Could you check a few things on this model? Use its own coordinates, in mm. A direction names the side the tool comes from. Round coordinates to 2 decimals unless told otherwise and drop trailing zeros. Loops run counter-clockwise (first coordinate to the right, second up) from the corner with the lowest first, then second, coordinate; pieces in that order, holes last. Notation, with made-up numbers: (27.5, 7) -> (74.5, 7) arc R9 cw to (74.5, 16) -> close; hole circle Ø9 at (65, 42). An arc over 180 degrees is marked (long way). Use CSV: the item, a comma, the result in double quotes. Start each with the question number.
```python
from build123d import *

# Parameters (mm, degrees)
BOSS_EXTRUDE1_DEPTH = 3
SKETCH3_W           = 10.2
SKETCH3_H           = 3.2
SKETCH3_W_2         = 3.2
SKETCH3_H_2         = 10.2
SKETCH3_H_3         = 7.372217102
CUT_EXTRUDE1_DEPTH  = 4


with BuildPart() as part:
    # Sketch2 → Boss-Extrude1 (new body)
    with BuildSketch(Plane(origin=(0, 0, 0), x_dir=(1, 0, 0), z_dir=(0, 1, 0))):
        with BuildLine():
            Line((-74.222217102, -66.842990858), (55.172217102, -66.842990858))
            Line((55.172217102, -66.842990858), (55.172217102, 43.501443346))
            Line((55.172217102, 43.501443346), (41.872217102, 43.501443346))
            ThreePointArc((41.872217102, 43.501443346), (38.336683196, 42.036977252), (36.872217102, 38.501443346))
            Line((36.872217102, 38.501443346), (36.872217102, -48.842990858))
            ThreePointArc((36.872217102, -48.842990858), (35.407751008, -52.378524764), (31.872217102, -53.842990858))
            Line((31.872217102, -53.842990858), (-31.872217102, -53.842990858))
            ThreePointArc((-31.872217102, -53.842990858), (-35.407751008, -52.378524764), (-36.872217102, -48.842990858))
            Line((-36.872217102, -48.842990858), (-36.872217102, 38.501443346))
            ThreePointArc((-36.872217102, 38.501443346), (-38.336683196, 42.036977252), (-41.872217102, 43.501443346))
            Line((-41.872217102, 43.501443346), (-74.222217102, 43.501443346))
            Line((-74.222217102, 43.501443346), (-74.222217102, -66.842990858))
        make_face()
    extrude(amount=-BOSS_EXTRUDE1_DEPTH)

    # Sketch3 → Cut-Extrude1 (cut, through all)
    with BuildSketch(Plane(origin=(0, 0, 0), x_dir=(1, 0, 0), z_dir=(0, 1, 0))):
        with Locations((-69.222217102, -65.342990858)):
            Rectangle(SKETCH3_W, SKETCH3_H)
        with Locations((-53.672217102, 18.329226244)):
            Rectangle(SKETCH3_W_2, SKETCH3_H_2)
        with Locations((-53.672217102, -1.670773756)):
            Rectangle(SKETCH3_W_2, SKETCH3_H_2)
        with Locations((-30, -65.342990858)):
            Rectangle(SKETCH3_W, SKETCH3_H)
        with Locations((-10, -65.342990858)):
            Rectangle(SKETCH3_W, SKETCH3_H)
        with Locations((-53.672217102, 36.915334795)):
            Rectangle(SKETCH3_W_2, SKETCH3_H_3)
        with Locations((30, -65.342990858)):
            Rectangle(SKETCH3_W, SKETCH3_H)
        with Locations((-53.672217102, -41.670773756)):
            Rectangle(SKETCH3_W_2, SKETCH3_H_2)
        with Locations((-53.672217102, -21.670773756)):
            Rectangle(SKETCH3_W_2, SKETCH3_H_2)
        with Locations((-53.672217102, -60.256882307)):
            Rectangle(SKETCH3_W_2, SKETCH3_H_3)
        Polygon((52.072217102, -56.570773756), (52.072217102, -63.742990858), (44.9, -63.742990858), (44.9, -66.942990858), (55.272217102, -66.942990858), (55.272217102, -56.570773756), align=None)
        with Locations((53.672217102, -21.670773756)):
            Rectangle(SKETCH3_W_2, SKETCH3_H_2)
        with Locations((53.672217102, -41.670773756)):
            Rectangle(SKETCH3_W_2, SKETCH3_H_2)
        with Locations((10, -65.342990858)):
            Rectangle(SKETCH3_W, SKETCH3_H)
        with Locations((53.672217102, 18.329226244)):
            Rectangle(SKETCH3_W_2, SKETCH3_H_2)
        with Locations((53.672217102, -1.670773756)):
            Rectangle(SKETCH3_W_2, SKETCH3_H_2)
        with Locations((53.672217102, 36.915334795)):
            Rectangle(SKETCH3_W_2, SKETCH3_H_3)
        with Locations((-72.722217102, 28.329226244)):
            Rectangle(SKETCH3_W_2, SKETCH3_H_2)
        with Locations((-72.722217102, 8.329226244)):
            Rectangle(SKETCH3_W_2, SKETCH3_H_2)
        with Locations((-72.722217102, -11.670773756)):
            Rectangle(SKETCH3_W_2, SKETCH3_H_2)
        with Locations((-69.222217102, 42.001443346)):
            Rectangle(SKETCH3_W, SKETCH3_H)
        with Locations((-64.622217102, -53.542990858)):
            Rectangle(SKETCH3_W_2, SKETCH3_H_2)
        with Locations((-64.622217102, 30.201443346)):
            Rectangle(SKETCH3_W_2, SKETCH3_H_2)
        with Locations((-72.722217102, -51.670773756)):
            Rectangle(SKETCH3_W_2, SKETCH3_H_2)
        with Locations((-72.722217102, -31.670773756)):
            Rectangle(SKETCH3_W_2, SKETCH3_H_2)
    extrude(amount=-CUT_EXTRUDE1_DEPTH, mode=Mode.SUBTRACT)


solid = part.part
```
1. We'd pull the mould along Z, two halves only. Please class faces 1 (the face through (30, -1, 63.743)), 2 (the face through (4.9, -1, 65)), 3 (the face through (52.072, -1, 42)), 4 (the face through (-71.122, -1, 32)): pulls with the +Z half, pulls with the -Z half, needs draft (parallel to the pull), parting line crosses it, or undercut.
2. Suppose I cut it at A-A (z = 3). List the corners of the cut face in (x, y) for me.
3. Suppose I cut it at C-C (x = 0). List the corners of the cut face in (y, z) for me, then the cut area to 3 significant figures.
4. Will these pins go through, and if not, where does the flat tip stop? pin 1 (1.5 mm diameter, centred on x = -13, y = -2.5, fed in from +Z); pin 2 (0.9 mm diameter, centred on y = -1.5, z = 0.5, fed in from +X); pin 3 (0.9 mm diameter, centred on x = -65, y = -1, fed in from -Z).
5. Suppose I cut it at B-B (y = -1.8). State how many separate pieces and enclosed holes the cut face has, then the cut area to 3 significant figures.
6. For faces 5 (the face through (-63.022, -1, -30)), 6 (the face through (-73, -1, -3.229)), 7 (the face through (54, -1, 16.571)), which set-ups out of +Z, -Z, +X, -X, +Y, -Y let a thin tool reach every point of the face, with its end or its side?
7. If I drill on L1, parallel to X at y = -0.4, z = -17.5; L2, parallel to X at y = -0.6, z = -26.5; L3, parallel to X at y = -0.9, z = 34.5, over which ranges is the centre line in solid material (lowest first)?
Geometry check:
1,face 1,"pulls with the +Z half"
1,face 2,"needs draft"
1,face 3,"undercut"
1,face 4,"undercut"
2,outline,"(-74.22, -3) -> (-55.27, -3) -> (-55.27, 0) -> (-74.22, 0) -> close; (-52.07, -3) -> (-36.87, -3) -> (-36.87, 0) -> (-52.07, 0) -> close; (36.87, -3) -> (52.07, -3) -> (52.07, 0) -> (36.87, 0) -> close"
3,outline,"(-3, 53.84) -> (0, 53.84) -> (0, 66.84) -> (-3, 66.84) -> close"
3,area,"39.0 mm²"
4,pin 1,"stops at z = 63.74"
4,pin 2,"stops at x = 52.07"
4,pin 3,"stops at z = -40.4"
5,separate pieces,"1"
5,enclosed holes,"8"
5,area,"6,310 mm²"
6,face 5,"+Y, -Y"
6,face 6,"-X, +Y, -Y"
6,face 7,"+X, +Y, -Y"
7,L1,"x = -74.22 to -55.27, -52.07 to -36.87, 36.87 to 52.07"
7,L2,"x = -71.12 to -66.22, -63.02 to -36.87, 36.87 to 55.17"
7,L3,"x = -71.12 to -36.87, 36.87 to 55.17"
